CAD build for the part. Positions are in the model's coordinates, mm. A direction names the side the tool comes from. Give positions to 0.01 mm unless a question says otherwise; leave off trailing zeros. Loops run counter-clockwise (first coordinate to the right, second up) from the corner with the lowest first, then second, coordinate; pieces in that order, holes last. Notation, with made-up numbers: M -5,-39 L 42,-39 A32 ccw 42,-9 Z; hole C -38.5,-38 d5. An arc over 180 degrees is marked long. Answer as CSV lines item,"result".
Autodesk Inventor part; units mm, degrees
ref_plane "Work Plane1" through (9.525, 162.8719, -37.7164) normal (0, 0, 1) x (1, 0, 0)
ref_plane "Work Plane3" through (19.05, 80.3219, 25.4) normal (0, 1, 0) x (-1, 0, 0)
ref_plane "Work Plane4" through (0, 228.9119, -25.0164) normal (0, 1, 0) x (-1, 0, 0)
sketch "Sketch1" plane through (0, 0, 0) normal (0, 0, 1) x (1, 0, 0)
  arc A0 (19.05, 80.3219) -> (-19.05, 80.3219) centre (0, 0) ccw
  line L0 (0, 0) -> (0, 152.4) construction
  line L1 (0, 93.0219) -> (19.05, 93.0219)
  line L2 (19.05, 93.0219) -> (19.05, 80.3219)
  line L3 (0, 93.0219) -> (-19.05, 93.0219)
  line L4 (-19.05, 93.0219) -> (-19.05, 80.3219)
  dimension "telescopeTubeDiameter" = 165.1
  dimension "d1" = 152.4
  dimension "d2" = 19.05
  dimension "d3" = 12.7
extrude "Extrusion1" add sketch "Sketch1" along normal mid plane 50.8
sketch "Sketch2" plane through (-19.05, 93.0219, 25.4) normal (0, 1, 0) x (1, 0, 0)
  line L0 (38.1, 0) -> (0, 0) construction
  line L1 (19.05, 0) -> (19.05, 50.8) construction
  line L2 (0, 50.8) -> (38.1, 50.8) construction
  line L3 (0, 50.8) -> (0, 0) construction
  line L4 (0, 25.4) -> (38.1, 25.4) construction
  line L5 (38.1, 50.8) -> (38.1, 0) construction
  line L6 (29.21, 19.05) -> (29.21, 31.75) construction
  line L7 (31.75, 19.05) -> (31.75, 31.75)
  line L8 (26.67, 31.75) -> (26.67, 19.05)
  arc A0 (26.67, 19.05) -> (31.75, 19.05) centre (29.21, 19.05) ccw
  arc A1 (31.75, 31.75) -> (26.67, 31.75) centre (29.21, 31.75) ccw
  point P0 (19.05, 25.4)
  point P1 (29.21, 25.4)
  dimension "d6" = 0
  dimension "d7" = 10.16
  dimension "d8" = 6.35
  dimension "d11" = 5.08
extrude "Extrusion2" cut sketch "Sketch2" against normal through all
mirror "Mirror1" about plane through (0, 0, 0) normal (1, 0, 0) of "Extrusion2"
sketch "Sketch3" plane through (0, 0, 0) normal (1, 0, 0) x (0, 1, 0)
  line L0 (93.0219, 25.4) -> (93.0219, -25.4)
  line L1 (80.3219, -25.4) -> (93.0219, -25.4)
  line L2 (162.8719, -25.4) -> (162.8719, -37.137) construction
  line L3 (93.0219, -25.4) -> (162.8719, -37.7164)
  line L4 (93.0219, -25.4) -> (162.8719, -25.4) construction
  line L5 (93.0219, -18.952) -> (162.8719, -31.2685)
  line L6 (162.8719, -31.2685) -> (162.8719, -37.7164)
  point P0 (0, 0)
  dimension "d13" = 69.85
  dimension "d14" = 10
  dimension "d15" = 6.35
extrude "Extrusion3" add sketch "Sketch3" along normal mid plane 19.05
ref_plane "Work Plane1" through (9.525, 162.8719, -37.7164) normal (0, 0, 1) x (1, 0, 0)
sketch "Sketch4" plane through (9.525, 162.8719, -37.7164) normal (0, 0, 1) x (1, 0, 0)
  line L0 (0, 0) -> (-19.05, 0)
  line L1 (-19.05, 0) -> (0, 0) construction
  line L2 (-9.525, 0) -> (-9.525, 50.8) construction
  circle A0 centre (-9.525, 44.45) radius 15.24
  arc A1 (0, 25.0747) -> (-19.05, 25.0747) centre (-9.525, 44.45) ccw
  line L3 (0, 0) -> (0, 25.0747)
  line L4 (-19.05, 0) -> (-19.05, 25.0747)
  point P0 (-9.525, -162.8719)
  dimension "d18" = 50.8
  dimension "d19" = 30.48
  dimension "d20" = 6.35
  dimension "d25" = 44.45
extrude "Extrusion4" add sketch "Sketch4" along normal blind 12.7
sketch "Sketch7" plane through (0, 0, 0) normal (1, 0, 0) x (0, 1, 0)
  line L0 (93.0219, -18.952) -> (162.8719, -31.2685)
  line L1 (162.8719, -31.2685) -> (162.8719, -25.0164)
  line L2 (162.8719, -25.0164) -> (127.4148, -25.0164)
  line L3 (127.4148, -25.0164) -> (162.8719, -31.2685)
  line L4 (187.9465, -25.0164) -> (162.8719, -25.0164)
  line L5 (162.8719, -31.2685) -> (162.8719, -25.0164)
  point P0 (0, 0)
extrude "Extrusion5" add sketch "Sketch7" along normal mid plane 19.05
mirror "Mirror4" about plane through (0, 0, 0) normal (0, 0, 1) of "Extrusion4", "Extrusion3"
sketch "Sketch8" plane through (0, 0, 0) normal (1, 0, 0) x (0, 1, 0)
  line L0 (162.8719, 31.2685) -> (162.8719, 25.0164)
  line L1 (93.0219, 18.952) -> (162.8719, 31.2685)
  line L2 (162.8719, 25.0164) -> (127.4148, 25.0164)
  line L3 (127.4148, 25.0164) -> (162.8719, 31.2685)
  line L4 (162.8719, 31.2685) -> (162.8719, 25.0164)
  point P0 (0, 0)
extrude "Extrusion6" add sketch "Sketch8" along normal mid plane 19.05
ref_plane "Work Plane3" through (19.05, 80.3219, 25.4) normal (0, 1, 0) x (-1, 0, 0)
ref_plane "Work Plane4" through (0, 228.9119, -25.0164) normal (0, 1, 0) x (-1, 0, 0)
equation "\"d62\" = 0.125 * Sketch12_Pitch"
equation "\"Sketch12_Pitch\" = 0.79375"
equation "\"d64\" = 60deg"
equation "\"d101\" = 55deg"
equation "\"Sketch15_Pitch\" = 0.79375"
equation "\"d119\" = 55deg"
equation "\"Sketch17_Pitch\" = 0.79375"
equation "\"d137\" = 55deg"
equation "\"Sketch19_Pitch\" = 0.79375"
equation "\"d155\" = 55deg"
equation "\"Sketch21_Pitch\" = 0.79375"
equation "\"d173\" = 55deg"
equation "\"Sketch23_Pitch\" = 0.79375"
equation "\"d191\" = 55deg"
equation "\"Sketch25_Pitch\" = 0.79375"
properties part number "finderV02"
Q1. Cut at A-A (z = -3.5). Write the cut outline in (x, y).
Solution:
outline,"M -19.05,80.32 A82.55 cw -12.7,81.57 L -12.7,93.02 L -19.05,93.02 Z; M -7.62,82.2 A82.55 cw 7.62,82.2 L 7.62,93.02 L -7.62,93.02 Z; M 12.7,81.57 A82.55 cw 19.05,80.32 L 19.05,93.02 L 12.7,93.02 Z"
Q2. Cut at C-C (x = 0). Write the cut outline in (y, z), and give its area (3 significant figures).
Solution:
outline,"M 82.55,-25.4 L 93.02,-25.4 L 162.87,-37.72 L 192.08,-37.72 L 192.08,-25.02 L 127.41,-25.02 L 93.02,-18.95 L 93.02,18.95 L 127.41,25.02 L 192.08,25.02 L 192.08,37.72 L 162.87,37.72 L 93.02,25.4 L 82.55,25.4 Z; M 222.56,-37.72 L 228.91,-37.72 L 228.91,-25.02 L 222.56,-25.02 Z; M 222.56,25.02 L 228.91,25.02 L 228.91,37.72 L 222.56,37.72 Z"
area,"2,560 mm²"
Q3. Wall check: line 1 (Z direction, x = -5.5, y = 172); line 2 (X direction, y = 115, z = -25.5) (3 decimals); line 3 (Y direction, x = -19, z = -15). Give the ranges that are in metal, low to high. Write a range as [from, to].
Solution:
line 1,"z = [-37.72, -25.02], [25.02, 37.72]"
line 2,"x = [-9.525, 9.525]"
line 3,"y = [80.33, 93.02]"
Q4. Mould opens along X. For faces 1 (the flat face through (-9.525, 152, 28)), 2 (the flat face through (0, 179, 25.016)), 3 (the cylindrical face through (7.03, 193.8, 31.46)) say: released by +X, released by -X, zero draft, split by the parting line, or undercut.
Solution:
face 1,"released by -X"
face 2,"zero draft"
face 3,"undercut"
Q5. Which spindle directions (+Z, -Z, +X, -X, +Y, -Y) get a long thin tool onto all of the face, cutting with end or side? Do faces 4 (the flat face through (-12.7, 87, 0)), 5 (the flat face through (-0.133, 109.978, -21.942)), 6 (the flat face through (-9.525, 150, -28)). Say none if no direction does.
Solution:
face 4,"+Y, -Y"
face 5,"+X, -X, +Y"
face 6,"+Z, -Z, -X"
Q6. Cut at B-B (y = 183.5). Write the cut outline in (x, z) (3 decimals).
Solution:
outline,"M -9.525,-37.716 L 9.525,-37.716 L 9.525,-25.016 L -9.525,-25.016 Z; M -9.525,25.016 L 9.525,25.016 L 9.525,37.716 L -9.525,37.716 Z"
Q7. Cut at D-D (y = 96.5). Write the cut outline in (x, z) (3 decimals).
Solution:
outline,"M -9.525,-26.013 L 9.525,-26.013 L 9.525,-19.565 L -9.525,-19.565 Z; M -9.525,19.565 L 9.525,19.565 L 9.525,26.013 L -9.525,26.013 Z"
Q8. Pin check, flat tips, straight feed: P1, Ø5.5, axis at y = 87, z = 3, coming from the -X side; P2, Ø4, axis at x = -0.5, y = 88, coming from the +Z side; P3, Ø15, axis at y = 119.5, z = -24.5, coming from the +X side (3 decimals); P4, Ø24.5, axis at x = 0, y = 207.32, coming from the -Z side. Stop position of each tip, or through.
Solution:
P1,"stops at x = -19.05"
P2,"stops at z = 25.4"
P3,"stops at x = 9.525"
P4,"passes through"
